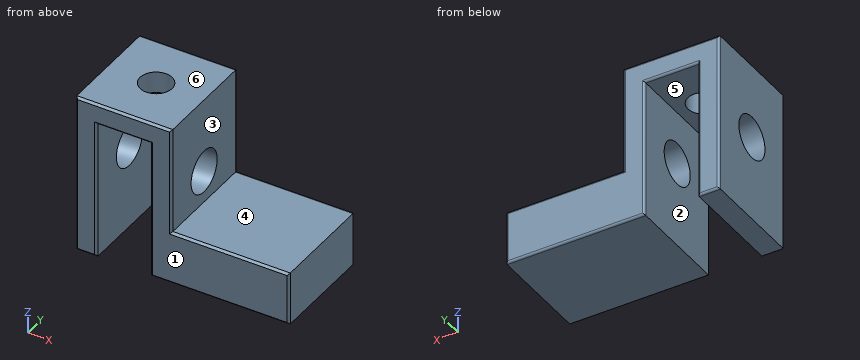
from build123d import *

# Parameters (mm, degrees)
F0_W     = 100
F0_H     = 50
F1_DEPTH = 25
F2_W     = 45
F2_H     = 50
F3_DEPTH = 50
F4_W     = 25
F4_H     = 65
F5_DEPTH = 50.001
F6_R     = 10
F7_DEPTH = 100.001
F8_R     = 7.5
F9_DEPTH = 10
F10_SIZE = 1
F11_R    = 1


with BuildPart() as f1:
    # F0 (on Top) → F1 (new body)
    with BuildSketch(Plane.XY):
        with Locations((50, 25)):
            Rectangle(F0_W, F0_H)
    extrude(amount=F1_DEPTH)

    # F2 (on face) → F3 (join)
    with BuildSketch(Plane.XY.offset(25)):
        with Locations((22.5, 25)):
            Rectangle(F2_W, F2_H)
    extrude(amount=F3_DEPTH)

    # F4 (on face) → F5 (cut, through all)
    with BuildSketch(Plane.XZ):
        with Locations((22.5, 32.5)):
            Rectangle(F4_W, F4_H)
    extrude(amount=-F5_DEPTH, mode=Mode.SUBTRACT)

    # F6 (on face) → F7 (cut, through all)
    with BuildSketch(Plane(origin=(0, 0, 0), x_dir=(0, -1, 0), z_dir=(-1, 0, 0))):
        with Locations((-25, 40)):
            Circle(F6_R)
    extrude(amount=-F7_DEPTH, mode=Mode.SUBTRACT)

    # F8 (on face) → F9 (cut, through all)
    with BuildSketch(Plane.XY.offset(75)):
        with Locations((22.5, 25)):
            Circle(F8_R)
    extrude(amount=-F9_DEPTH, mode=Mode.SUBTRACT)

    # F10
    f10_edges = [f1.edges().sort_by_distance(p)[0] for p in [
        (0, 0, 37.5),
        (35, 0, 32.5),
        (22.5, 0, 65),
        (5, 0, 0),
        (10, 0, 32.5),
        (67.5, 0, 0),
        (100, 0, 12.5),
        (72.5, 0, 25),
        (45, 0, 50),
        (22.5, 0, 75),
    ]]
    chamfer(f10_edges, length=F10_SIZE)

    # F11
    f11_edges = [f1.edges().sort_by_distance(p)[0] for p in [
        (72.5, 50, 25),
        (45, 50, 50),
        (22.5, 50, 75),
        (0, 50, 37.5),
        (67.5, 50, 0),
        (35, 50, 32.5),
        (22.5, 50, 65),
        (10, 50, 32.5),
        (5, 50, 0),
        (100, 50, 12.5),
    ]]
    fillet(f11_edges, radius=F11_R)


solid = f1.part
Can you work these out from the model? Positions are in its coordinate system, mm. Face numbers are marked on the shaded views. A direction names the side the tool comes from. Round coordinates to 2 decimals unless told otherwise and drop trailing zeros. Write each loop counter-clockwise with the first axis right and the second up, starting at its lowest first coordinate (ties: lowest second). Pieces come first, ordered by that corner, then holes. Notation, with made-up numbers: (32, 34.5) -> (54, 34.5) arc R27 cw to (54, 68.5) -> close; hole circle Ø10 at (1, -2). An arc over 180 degrees is marked (long way). Use one line per item in the form item = value. Start each with the question number.
Q1. Imagine slicing it at A-A (z = 57). Please give me the cut outline in (x, y).
Q2. I'm going to push flat-ended pins straight in: P1, Ø24, axis at x = 71, y = 36.5, coming from the +Z side; P2, Ø10, axis at y = 22, z = 46, coming from the +X side; P3, Ø24, axis at y = 34, z = 29.5, coming from the +X side; P4, Ø24, axis at x = 22.5, y = 25, coming from the -Z side. Where does each tip first touch, or does it pass through?
Q3. Imagine slicing it at C-C (y = 25). Please give me the cut outline in (x, z).
Q4. Which directions (+Z, -Z, +X, -X, +Y, -Y) give clear straight access to the entire face, cutting with the end or side of a thin tool? Please do the marked faces 4, 5 and 6.
Q5. Imagine slicing it at B-B (z = 40). Please give me the cut outline in (x, y), then the cut area to 3 significant figures.
Q6. We'd pull the mould along X, two halves only. Please class the marked faces 1, 2 and 3: +X half, -X half, draft (parallel to the pull), parting line (faces both ways), or undercut.
Q7. If I drill on probe 1 along X at (y, z) = (9, 56.5); probe 2 along Z at (x, y) = (4, 25); probe 3 along X at (y, z) = (15, 23), over which ranges is the centre line in solid material (lowest first)? Write a range as [from, to].
Q8. Imagine slicing it at D-D (x = 22.5). Please give me the cut outline in (y, z).
Worked out:
q1.outline = (0, 1) -> (1, 0) -> (9, 0) -> (10, 1) -> (10, 49) arc R1 ccw to (9, 50) -> (1, 50) arc R1 ccw to (0, 49) -> close; (35, 1) -> (36, 0) -> (44, 0) -> (45, 1) -> (45, 49) arc R1 ccw to (44, 50) -> (36, 50) arc R1 ccw to (35, 49) -> close
q2.P1 = 25
q2.P2 = 45
q2.P3 = 100
q2.P4 = 65
q3.outline = (0, 0) -> (10, 0) -> (10, 30) -> (0, 30) -> close; (0, 50) -> (10, 50) -> (10, 65) -> (15, 65) -> (15, 75) -> (0, 75) -> close; (30, 65) -> (35, 65) -> (35, 50) -> (45, 50) -> (45, 75) -> (30, 75) -> close; (35, 0) -> (100, 0) -> (100, 25) -> (45, 25) -> (45, 30) -> (35, 30) -> close
q4.face_4 = +Z, +X, +Y, -Y
q4.face_5 = -Z, +Y, -Y
q4.face_6 = +Z, +X, -X, +Y, -Y
q5.outline = (0, 1) -> (1, 0) -> (9, 0) -> (10, 1) -> (10, 15) -> (0, 15) -> close; (0, 35) -> (10, 35) -> (10, 49) arc R1 ccw to (9, 50) -> (1, 50) arc R1 ccw to (0, 49) -> close; (35, 1) -> (36, 0) -> (44, 0) -> (45, 1) -> (45, 15) -> (35, 15) -> close; (35, 35) -> (45, 35) -> (45, 49) arc R1 ccw to (44, 50) -> (36, 50) arc R1 ccw to (35, 49) -> close
q5.area = 597 mm^2
q6.face_1 = draft
q6.face_2 = undercut
q6.face_3 = +X half
q7.probe_1 = [0, 10], [35, 45]
q7.probe_2 = [0, 30], [50, 75]
q7.probe_3 = [0, 10], [35, 100]
q8.outline = (0, 66) -> (1, 65) -> (17.5, 65) -> (17.5, 75) -> (1, 75) -> (0, 74) -> close; (32.5, 65) -> (49, 65) arc R1 ccw to (50, 66) -> (50, 74) arc R1 ccw to (49, 75) -> (32.5, 75) -> close
